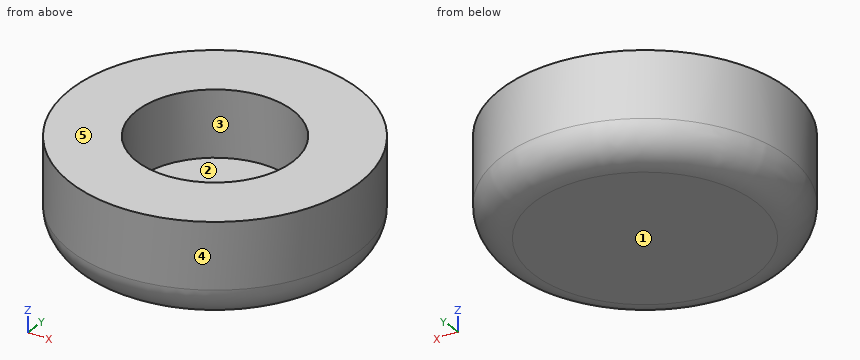
Autodesk Fusion 360 part; units mm, degrees
sketch "Sketch1" plane through (0, 0, 0) normal (0, 0, 1) x (1, 0, 0)
  circle A0 centre (0, 0) radius 3.55
  circle A1 centre (0, 0) radius 6.55
  dimension "d1" = 7.1
  dimension "d2" = 3
extrude "Extrude1" add sketch "Sketch1" along normal blind 3
extrude "Extrude3" add sketch "Sketch1" against normal blind 1.5 contours A0 | A1
fillet "Fillet1" radius 1.5 1 edges at (-6.1067, 2.3686, -1.5)
CAD build for the part. Positions are in the model's coordinates, mm. Face numbers are marked on the shaded views. A direction names the side the tool comes from. Coordinates: 2 decimals unless noted, no trailing zeros. Loops run counter-clockwise (first coordinate to the right, second up) from the corner with the lowest first, then second, coordinate; pieces in that order, holes last. Notation, with made-up numbers: (-24, -22) - (4, -22) arc R29 ccw to (4, 11) - close; hole circle Ø11 at (61.25, -8). An arc over 180 degrees is marked (long way). Use one line per item in the form item = value. Start each with the question number.
1) Flat gauge pins, fed straight in: pin 1 (2 mm diameter, centred on y = 5, z = -0.5, fed in from -X); pin 2 (1.5 mm diameter, centred on y = -4.5, z = 1, fed in from -X); pin 3 (3.5 mm diameter, centred on x = -1.5, y = 0, fed in from +Z). Where does each tip first touch, or does it go through?
2) Band-saw the part on A-A (x = 0). Give the cut face in (y, z).
3) Tool access for the marked faces 1 and 2: list every direction of +Z, -Z, +X, -X, +Y, -Y with a clear straight run to the whole face (end or side of a thin tool).
4) Band-saw the part on C-C (z = 2.7). Give the cut face in (x, y).
5) Drill centre lines: L1, parallel to Y at x = 0, z = 0.75; L2, parallel to Z at x = -2, y = -2; L3, parallel to X at y = 0.25, z = 1.45. Where is each one in solid material? Low to high. Write a range as from..to.
6) Band-saw the part on D-D (z = -0.6). Give the cut face in (x, y), and give its area (3 significant figures).
7) Two-plate mould, pull along X, no slides. Class the marked faces 3, 4 and 5: +X half, -X half, draft (parallel to the pull), parting line (faces both ways), or undercut.
Check values:
q1.pin_1 = -5.14
q1.pin_2 = -5.37
q1.pin_3 = 0
q2.outline = (-6.55, 0) arc R1.5 ccw to (-5.05, -1.5) - (5.05, -1.5) arc R1.5 ccw to (6.55, 0) - (6.55, 3) - (3.55, 3) - (3.55, 0) - (-3.55, 0) - (-3.55, 3) - (-6.55, 3) - close
q3.face_1 = -Z, +X, -X, +Y, -Y
q3.face_2 = +Z
q4.outline = circle Ø13.1 at (0, 0); hole circle Ø7.1 at (0, 0)
q5.L1 = -6.55..-3.55, 3.55..6.55
q5.L2 = -1.5..0
q5.L3 = -6.55..-3.54, 3.54..6.55
q6.outline = circle Ø12.85 at (0, 0)
q6.area = 130 mm2
q7.face_3 = undercut
q7.face_4 = parting line
q7.face_5 = draft
